Read the model definition and answer for the solid it produces. Units are mm, in the model's axes. Face numbers are marked on the shaded views. Coordinates: 2 decimals unless noted, no trailing zeros. Write each loop counter-clockwise with the first axis right and the second up, starting at its lowest first coordinate (ties: lowest second). Pieces come first, ordered by that corner, then holes.
(1) Find the intervals of material crossed by probe 1 along X at (y, z) = (0, 6); probe 2 along Y at (x, z) = (-0.25, 9); probe 3 along Y at (x, z) = (-2.25, 9.75), in increasing order.
(2) Section D-D on z = 4.5 is taken. Write down the section's boundary in (x, y).
(3) Section C-C on y = -3.5 is taken. Write down the section's boundary in (x, z), then the cut area to 3 significant figures.
(4) Section A-A on z = 8 is taken. Write down the section's boundary in (x, y), then the cut area to 3 significant figures.
(5) Given pin 1 (4 mm diameter, centred on y = -2.5, z = 4.5, fed in from +X); pin 2 (1 mm diameter, centred on x = 3, z = 5.5, fed in from +Y); pin 3 (5 mm diameter, centred on y = 3.5, z = 3.5, fed in from -X); pin 4 (3 mm diameter, centred on x = -0.5, z = 3, fed in from +Y), each flat-ended and moving along its own axis, determine where each tip first touches the part or whether it passes through.
(6) Section B-B on x = 2 is taken. Write down the section's boundary in (y, z).
(7) The mould has two halves that part along X. Classify the marked faces 1, 2 and 3: +X half, -X half, draft (parallel to the pull), parting line (faces both ways), or undercut.
from build123d import *

# Parameters (mm, degrees)
F0_R          = 5
F1_DEPTH      = 10
F3_DEPTH      = 5.001
F3_DEPTH_BACK = 5.001
F5_DEPTH      = 5.0010001
F5_DEPTH_BACK = 5.0010001
F6_R          = 4
F7_DEPTH      = 10.0010001


with BuildPart() as f1:
    # F0 (on Top) → F1 (new body)
    with BuildSketch(Plane.XY):
        Circle(F0_R)
    extrude(amount=F1_DEPTH)

    # F2 (on Front) → F3 (cut, two sides)
    with BuildSketch(Plane.XZ) as f3_sk:
        with BuildLine():
            ThreePointArc((4, 0), (0, 4), (-4, 0))
            Line((-4, 0), (4, 0))
        make_face()
    extrude(amount=-F3_DEPTH, mode=Mode.SUBTRACT)
    extrude(f3_sk.sketch, amount=F3_DEPTH_BACK, mode=Mode.SUBTRACT)

    # F4 (on Right) → F5 (cut, two sides)
    with BuildSketch(Plane.YZ) as f5_sk:
        with BuildLine():
            ThreePointArc((-4, 10), (0, 6.0994715953), (4, 10))
            Line((4, 10), (-4, 10))
        make_face()
    extrude(amount=-F5_DEPTH, mode=Mode.SUBTRACT)
    extrude(f5_sk.sketch, amount=F5_DEPTH_BACK, mode=Mode.SUBTRACT)

    # F6 (on Top) → F7 (cut, through all)
    with BuildSketch(Plane.XY):
        Circle(F6_R)
    extrude(amount=F7_DEPTH, mode=Mode.SUBTRACT)


solid = f1.part
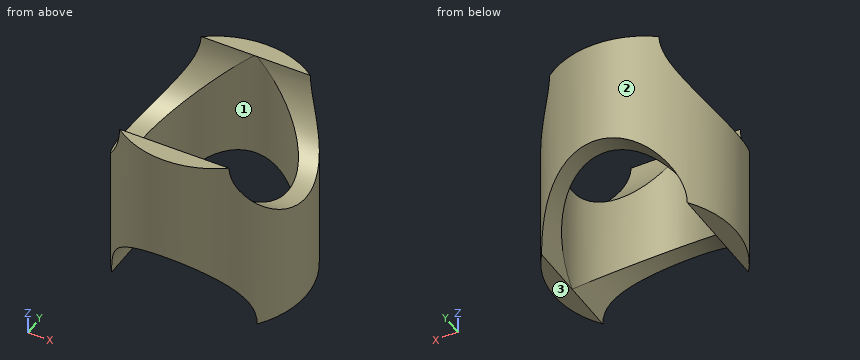
Response:
1. probe 1: x = -5 to -4, 4 to 5
1. probe 2: y = -4.99 to -3.99, 3.99 to 4.99
1. probe 3: y = -4.47 to -3.99, 3.99 to 4.47
2. outline: circle Ø10 at (0, 0); hole circle Ø8 at (0, 0)
3. outline: (-3.57, 1.8) arc R4 cw to (-1.94, 3.5) - (-1.94, 8.16) - (-3.57, 8.16) - close; (1.94, 3.5) arc R4 cw to (3.57, 1.8) - (3.57, 8.16) - (1.94, 8.16) - close
3. area: 17.5 mm2
4. outline: (-3.66, -3.41) arc R5 ccw to (3.66, -3.41) - (2.1, -3.41) arc R4 cw to (-2.1, -3.41) - close; (-3.66, 3.41) - (-2.1, 3.41) arc R4 cw to (2.1, 3.41) - (3.66, 3.41) arc R5 ccw to start
4. area: 12.8 mm2
5. pin 1: stops at x = 4.97
5. pin 2: stops at y = 4.33
5. pin 3: stops at x = -4.9
5. pin 4: stops at y = 5
6. outline: (-4.58, 3.46) - (-3.46, 3.46) - (-3.46, 8.1) arc R4 cw to (-4, 10) - (-4.58, 10) - close; (3.46, 3.46) - (4.58, 3.46) - (4.58, 10) - (4, 10) arc R4 cw to (3.46, 8.1) - close
7. face 1: undercut
7. face 2: parting line
7. face 3: draft
